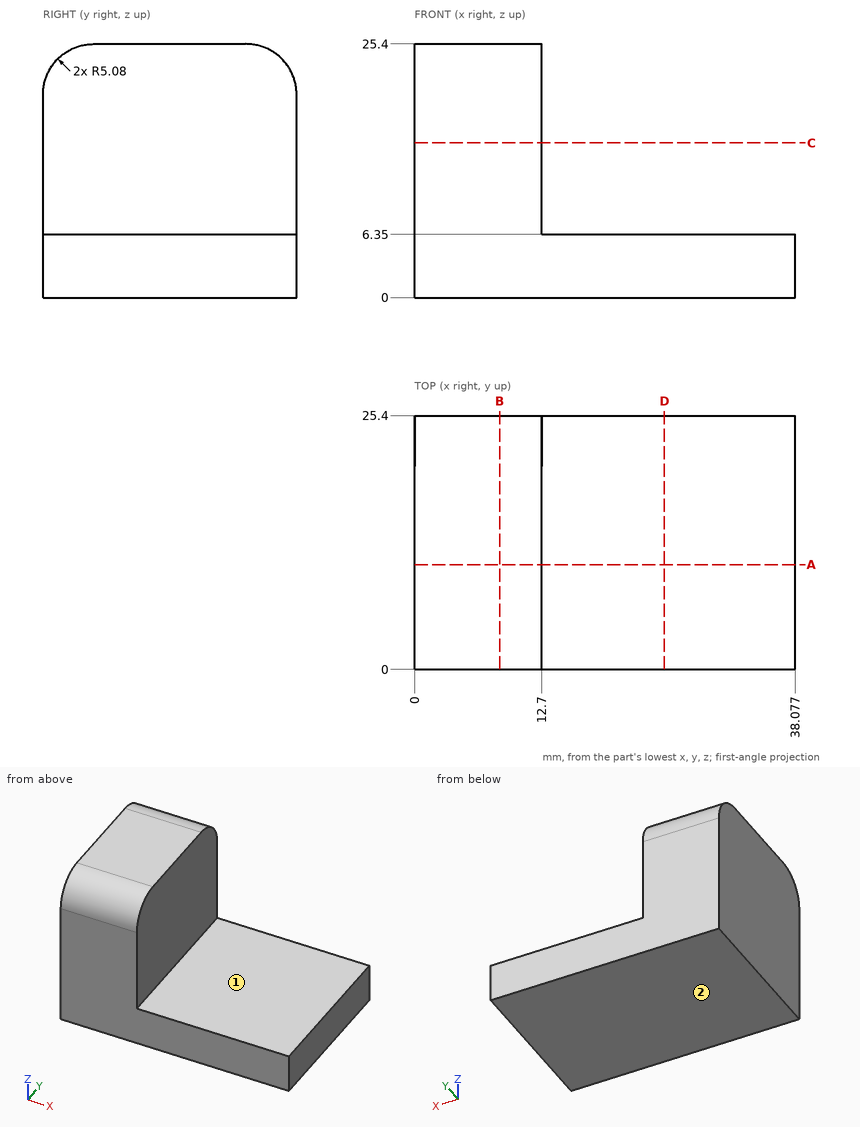
For this review, use the dimensioned drawing (mm, ordinates from the lowest corner) and the shaded views. A direction names the side the tool comes from. Give positions to 0.01 mm unless a question says otherwise; leave off trailing zeros. Loops run counter-clockwise (first coordinate to the right, second up) from the corner with the lowest first, then second, coordinate; pieces in that order, holes last.
Item 1: Take a section at B-B, the plane x = 8.5. State the section outline as (y, z) points.
Item 2: Take a section at A-A, the plane y = 10.5. State the section outline as (x, z) points.
Item 3: Insertion check: pin 1 (9.5 mm diameter, centred on y = 11.5, z = 12, fed in from +X); pin 2 (3 mm diameter, centred on x = 15.5, y = 16, fed in from +Z). Each pin has a flat end and moves straight along its axis. Give the tip position at first contact, or say it passes through.
Item 4: Tool access review of the marked faces 1 and 2: name each direction out of +Z, -Z, +X, -X, +Y, -Y from which nothing blocks a thin tool from reaching the whole face with its end or side.
Item 5: Take a section at D-D, the plane x = 25. State the section outline as (y, z) points, and give its area (3 significant figures).
Item 6: Take a section at C-C, the plane z = 15.5. State the section outline as (x, y) points.
Item 7: For line 1 along X through (y, z) = (16.75, 12.5); line 2 along Z through (x, y) = (20, 11.5); line 3 along Z through (x, y) = (11, 22.5), list the stretches that pass through material, from the lowest coordinate up.
Calculated:
1. outline: (0, 0) - (25.4, 0) - (25.4, 20.32) arc R5.08 ccw to (20.32, 25.4) - (5.08, 25.4) arc R5.08 ccw to (0, 20.32) - close
2. outline: (0, 0) - (38.08, 0) - (38.08, 6.35) - (12.7, 6.35) - (12.7, 25.4) - (0, 25.4) - close
3. pin 1: stops at x = 12.7
3. pin 2: stops at z = 6.35
4. face 1: +Z, +X, +Y, -Y
4. face 2: -Z, +X, -X, +Y, -Y
5. outline: (0, 0) - (25.4, 0) - (25.4, 6.35) - (0, 6.35) - close
5. area: 161 mm2
6. outline: (0, 0) - (12.7, 0) - (12.7, 25.4) - (0, 25.4) - close
7. line 1: x = 0 to 12.7
7. line 2: z = 0 to 6.35
7. line 3: z = 0 to 24.91
